Input: part model. Units: mm. Frame: model coordinates. Face numbers are marked on the shaded views. A direction names the side the tool comes from. Round coordinates to 2 decimals unless told otherwise and drop trailing zeros. Order: outer loops, then holes, each group sorted by start corner. A loop starts at its lowest first (then second) coordinate and runs counter-clockwise, first axis right, second up. Notation, with made-up numbers: (-36, -8.5) -> (-7, -8.5) arc R30 ccw to (-7, 13.5) -> close; hole circle Ø1 at (84, 29.5). An arc over 180 degrees is marked (long way). Answer as CSV lines item,"result". Start each with the question number.
1) Mould query, pull axis Z, two halves, no side actions, for the marked faces 1 and 2. Classes: +Z half, -Z half, draft (parallel to the pull), parting line (faces both ways), or undercut.
2) Section query B-B, the plane y = 1.5. Output: boundary loops of the cut face in (x, z).
3) Access query for the marked faces 3 and 4. Directions: +Z, -Z, +X, -X, +Y, -Y. A direction counts if a zero-diameter tool reaches every point of the face in a straight line with its end or side. Return the directions, or none.
4) First-contact query: P1, Ø1.5, axis at x = 6, z = -3, coming from the -Y side; P2, Ø18.5, axis at y = 0, z = 0, coming from the -X side; P3, Ø6, axis at x = 11.5, y = -9.5, coming from the -Z side; P4, Ø2, axis at x = -0.5, y = -5.5, coming from the -Z side. Flat tips, straight axial feed; report the tip coordinate or a pass-through.
5) Line query: L1, parallel to Z at x = -18, y = 0; L2, parallel to Y at x = 10, z = 0; L3, parallel to Z at x = 2, y = 1.5. Output: solid intervals per line, ascending.
6) Section query D-D, the plane y = 10.5. Output: boundary loops of the cut face in (x, z).
7) Section query A-A, the plane z = 0. Output: boundary loops of the cut face in (x, y).
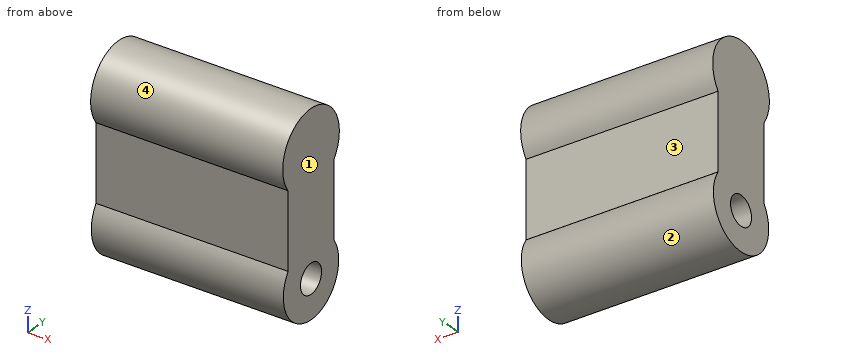
```python
from build123d import *

# Parameters (mm, degrees)
F0_R      = 15.2590123091
F1_DEPTH  = 38.1
F2_R      = 15.2230009986
F3_DEPTH  = 38.1
F4_DEPTH  = 38.1
F5_R      = 5.7970775931
F6_DEPTH  = 50.8
F7_DEPTH  = 101.6
F10_DEPTH = 38.1
F11_DEPTH = 38.1
F12_R     = 15.6063789954
F13_DEPTH = 38.1
F14_DEPTH = 38.1
F15_DEPTH = 38.1


with BuildPart() as f1:
    # F0 (on Right) → F1 (new body)
    with BuildSketch(Plane.YZ):
        Circle(F0_R)
    extrude(amount=F1_DEPTH)

    # F2 (on Right) → F3 (join)
    with BuildSketch(Plane.YZ):
        Circle(F2_R)
    extrude(amount=F3_DEPTH)

    # F2 (on Right) → F4 (join)
    with BuildSketch(Plane.YZ):
        Circle(F2_R)
    extrude(amount=-F4_DEPTH)

    # F5 (on Right) → F6 (join)
    with BuildSketch(Plane.YZ):
        Circle(F5_R)
    extrude(amount=-F6_DEPTH)

    # F7 (cut): a face of the model
    f7_faces = [f1.faces().sort_by_distance(p)[0] for p in [
        (-50.8, 0, 0),
    ]]
    extrude(f7_faces, amount=-F7_DEPTH, mode=Mode.SUBTRACT)

    # F9 (on Right) → F10 (join)
    with BuildSketch(Plane.YZ):
        Polygon((-12.7270547673, 38.6252403259), (-12.6615641639, 8.5206106305), (12.6757137477, 8.5206106305), (12.6757137477, 38.6252403259), align=None)
    extrude(amount=F10_DEPTH)

    # F11 (add): a face of the model
    f11_faces = [f1.faces().sort_by_distance(p)[0] for p in [
        (0, -0.0109795031, 25.7338348124),
    ]]
    extrude(f11_faces, amount=F11_DEPTH)

    # F12 (on Right) → F13 (join)
    with BuildSketch(Plane.YZ):
        with Locations((0, 47.4579036236)):
            Circle(F12_R)
    extrude(amount=F13_DEPTH)

    # F14 (add): a face of the model
    f14_faces = [f1.faces().sort_by_distance(p)[0] for p in [
        (0, 0.0002381193, 49.6663951718),
    ]]
    extrude(f14_faces, amount=-F14_DEPTH)

    # F15 (add): a face of the model
    f15_faces = [f1.faces().sort_by_distance(p)[0] for p in [
        (0, 0.0002381193, 49.6663951718),
    ]]
    extrude(f15_faces, amount=F15_DEPTH)


solid = f1.part
```
Findings:
1,face 1,"draft"
1,face 2,"undercut"
2,outline,"(-38.1, -15.19) -> (38.1, -15.19) -> (38.1, -5.6) -> (-38.1, -5.6) -> close; (-38.1, 5.6) -> (38.1, 5.6) -> (38.1, 62.99) -> (-38.1, 62.99) -> close"
3,face 3,"+X, -X, +Y"
3,face 4,"+X, -X"
4,P1,"stops at y = -15.09"
4,P2,"stops at x = -38.1"
4,P3,"stops at z = -13.81"
4,P4,"stops at z = -14.58"
5,L1,"z = -15.26 to -5.8, 5.8 to 63.06"
5,L2,"y = -15.26 to -5.8, 5.8 to 15.26"
5,L3,"z = -15.19 to -5.6, 5.6 to 62.99"
6,outline,"(-38.1, -11.07) -> (38.1, -11.07) -> (38.1, 59) -> (-38.1, 59) -> close"
7,outline,"(-38.1, -15.26) -> (38.1, -15.26) -> (38.1, -5.8) -> (-38.1, -5.8) -> close; (-38.1, 5.8) -> (38.1, 5.8) -> (38.1, 15.26) -> (-38.1, 15.26) -> close"
